Geometry: final body of the model. Coordinates: model frame, mm. Face numbers are marked on the shaded views. A direction names the side the tool comes from. Give positions to 0.01 mm unless a question says otherwise; leave off trailing zeros. Order: outer loops, then holes, each group sorted by start corner. A loop starts at its lowest first (then second) coordinate and runs counter-clockwise, first axis right, second up. Notation, with made-up numbers: M 16.5,38 L 74.5,38 A14 ccw 74.5,49 Z; hole C 10,-37 d2. An arc over 180 degrees is marked long. One line per item, written item: value. Start each with the question number.
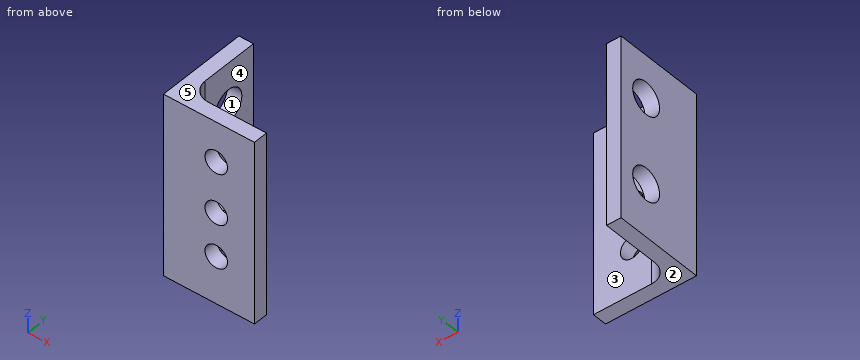
```python
from build123d import *

# Parameters (mm, degrees)
BOSS_EXTRUDE1_DEPTH = 12.7
SKETCH3_R           = 0.7874
CUT_EXTRUDE1_DEPTH  = 2.54
FILLET1_R           = 1.27
CUT_EXTRUDE2_REACH  = 3.016
SKETCH4_R           = 1.1303


with BuildPart() as part:
    # Sketch1 → Boss-Extrude1 (new body)
    with BuildSketch(Plane.XY):
        Polygon((-6.35, 6.35), (-6.35, 0), (0, 0), (0, 1.016), (-5.334, 1.016), (-5.334, 6.35), align=None)
    extrude(amount=BOSS_EXTRUDE1_DEPTH)

    # Sketch3 → Cut-Extrude1 (cut)
    with BuildSketch(Plane(origin=(0, 1.016, 0), x_dir=(1, 0, 0), z_dir=(0, 1, 0))):
        with Locations((-2.667, -9.906)):
            Circle(SKETCH3_R)
        with Locations((-2.667, -6.35)):
            Circle(SKETCH3_R)
        with Locations((-2.667, -3.302)):
            Circle(SKETCH3_R)
    extrude(amount=-CUT_EXTRUDE1_DEPTH, mode=Mode.SUBTRACT)

    # Fillet1
    fillet1_edges = [part.edges().sort_by_distance(p)[0] for p in [
        (-5.334, 1.016, 6.35),
    ]]
    fillet(fillet1_edges, radius=FILLET1_R)

    # Sketch4 → Cut-Extrude2 (cut, up to next)
    with BuildSketch(Plane(origin=(-5.334, 0, 0), x_dir=(0, 0, -1), z_dir=(1, 0, 0)), mode=Mode.PRIVATE) as cut_extrude2_sk1:
        with Locations((-9.7, 4.24)):
            Circle(SKETCH4_R)
    cut_extrude2_tool1 = extrude(cut_extrude2_sk1.sketch, amount=-CUT_EXTRUDE2_REACH, mode=Mode.PRIVATE) & part.part
    add(cut_extrude2_tool1.solids().sort_by_distance((-5.334, 4.24, 9.7))[0], mode=Mode.SUBTRACT)
    # Sketch4 → Cut-Extrude2 (cut, up to next)
    with BuildSketch(Plane(origin=(-5.334, 0, 0), x_dir=(0, 0, -1), z_dir=(1, 0, 0)), mode=Mode.PRIVATE) as cut_extrude2_sk2:
        with Locations((-3.7, 4.24)):
            Circle(SKETCH4_R)
    cut_extrude2_tool2 = extrude(cut_extrude2_sk2.sketch, amount=-CUT_EXTRUDE2_REACH, mode=Mode.PRIVATE) & part.part
    add(cut_extrude2_tool2.solids().sort_by_distance((-5.334, 4.24, 3.7))[0], mode=Mode.SUBTRACT)


solid = part.part
```
Q1. Ray query, line 1 along Z through (x, y) = (-2.5, 0.5); line 2 along X through (y, z) = (2.25, 8.5); line 3 along Y through (x, z) = (-2, 8.5). Return the intervals inside material, ascending. Write a range as [from, to].
Q2. Section query C-C on z = 9.7. Return loops of the section in (x, y), and give its area (3 significant figures).
Q3. Section query D-D on x = -3. Return loops of the section in (y, z).
Q4. Mould query, pull axis Y, two halves, no side actions, for the marked faces 1, 2 and 3. Classes: +Y half, -Y half, draft (parallel to the pull), parting line (faces both ways), or undercut.
Q5. Set-up query: the marked faces 4 and 5. Return all of +Z, -Z, +X, -X, +Y, -Y with unobstructed straight access to the full face (end or side cutting, diameter ignored); none if empty.
Q6. Section query B-B on z = 6.35. Return loops of the section in (x, y).
Q7. Section query A-A on y = 4.5. Return loops of the section in (x, z), and give its area (3 significant figures).
Q8. Contact query for flat-ended pins moving along their axis: pin 1 (2.5 mm diameter, centred on y = 4.24, z = 9.7, fed in from +X); pin 2 (3.5 mm diameter, centred on x = -2, z = 7, fed in from +Y); pin 3 (0.9 mm diameter, centred on x = -2.667, z = 6.35, fed in from -Y). Output: stop coordinate, or through.
Results below:
1. line 1: [0, 2.53], [4.07, 5.58], [7.12, 9.14], [10.68, 12.7]
1. line 2: [-6.35, -5.33]
1. line 3: [0, 1.02]
2. outline: M -6.35,0 L -3.43,0 L -3.43,1.02 L -4.06,1.02 A1.27 cw -5.33,2.29 L -5.33,3.11 L -6.35,3.11 Z; M -6.35,5.37 L -5.33,5.37 L -5.33,6.35 L -6.35,6.35 Z; M -1.91,0 L 0,0 L 0,1.02 L -1.91,1.02 Z
2. area: 8.38 mm2
3. outline: M 0,0 L 1.02,0 L 1.02,2.59 L 0,2.59 Z; M 0,4.02 L 1.02,4.02 L 1.02,5.64 L 0,5.64 Z; M 0,7.06 L 1.02,7.06 L 1.02,9.19 L 0,9.19 Z; M 0,10.62 L 1.02,10.62 L 1.02,12.7 L 0,12.7 Z
4. face 1: undercut
4. face 2: draft
4. face 3: +Y half
5. face 4: +Z, -Z, +X, +Y
5. face 5: +Z, +X, -X, +Y, -Y
6. outline: M -6.35,0 L -3.45,0 L -3.45,1.02 L -4.06,1.02 A1.27 cw -5.33,2.29 L -5.33,6.35 L -6.35,6.35 Z; M -1.88,0 L 0,0 L 0,1.02 L -1.88,1.02 Z
7. outline: M -6.35,0 L -5.33,0 L -5.33,2.6 L -6.35,2.6 Z; M -6.35,4.8 L -5.33,4.8 L -5.33,8.6 L -6.35,8.6 Z; M -6.35,10.8 L -5.33,10.8 L -5.33,12.7 L -6.35,12.7 Z
7. area: 8.43 mm2
8. pin 1: x = -5.33
8. pin 2: y = 1.02
8. pin 3: through
